from build123d import *

# Parameters (mm, degrees)
BOSS_EXTRUDE1_DEPTH      = 4.7625
M3_CLEARANCE_HOLE1_D     = 3.4
F_7_0_7_DIAMETER_HOLE1_D = 7
SKETCH12_R               = 11.5
CUT_EXTRUDE1_DEPTH       = 2.5


with BuildPart() as part:
    # Sketch1 → Boss-Extrude1 (new body)
    with BuildSketch(Plane(origin=(0, 0, 0), x_dir=(1, 0, 0), z_dir=(0, 1, 0))):
        Polygon((70, 65), (70, 45), (90, 45), (90, 0), (0, 0), (0, 65), align=None)
    extrude(amount=BOSS_EXTRUDE1_DEPTH)

    # M3 Clearance Hole1 (through all)
    with Locations(Plane(origin=(0, 4.7625, 0), x_dir=(1, 0, 0), z_dir=(0, 1, 0))):
        with Locations((36.709, 5.709), (36.709, 36.709), (5.709, 36.709), (5.709, 5.709)):
            Hole(M3_CLEARANCE_HOLE1_D / 2)

    # Ø7.0 (7) Diameter Hole1 (through all)
    with Locations(Plane(origin=(0, 0, 0), x_dir=(-1, 0, 0), z_dir=(0, -1, 0))):
        with Locations((-21.209, 21.209)):
            Hole(F_7_0_7_DIAMETER_HOLE1_D / 2)

    # Sketch12 → Cut-Extrude1 (cut)
    with BuildSketch(Plane.XZ):
        with Locations(Location((21.209, -21.209, 0), (0, 0, 270))):
            Circle(SKETCH12_R)
    extrude(amount=-CUT_EXTRUDE1_DEPTH, mode=Mode.SUBTRACT)


solid = part.part
Can you work these out from the model? Positions are in its coordinate system, mm. A direction names the side the tool comes from. Round coordinates to 2 decimals unless told otherwise and drop trailing zeros. Order: outer loops, then holes, each group sorted by start corner. A loop starts at its lowest first (then second) coordinate and runs counter-clockwise, first axis right, second up. Notation, with made-up numbers: (72, 44.5) - (102, 44.5) arc R27 ccw to (102, 63.5) - close; hole circle Ø2 at (-11, 39.25). An arc over 180 degrees is marked (long way). Answer in a Markdown table with one row per item.
(1) For P1, Ø11.5, axis at x = 17, z = -24, coming from the -Y side, with a flat end and sliding along its axis, tell me the tip position at first contact or that it passes through.
From the geometry:
| item | result |
|---|---|
| P1 | stops at y = 2.5 |
(2) Suppose I cut it at D-D, the plane z = -30. Please give me the cut outline in (x, y).
From the geometry:
| item | result |
|---|---|
| outline | (0, 0) - (13.79, 0) - (13.79, 2.5) - (28.62, 2.5) - (28.62, 0) - (90, 0) - (90, 4.76) - (0, 4.76) - close |
(3) Please list where these lines run through material, in increasing order: L1, parallel to X at y = 1.2, z = -21.5; L2, parallel to X at y = 3.95, z = -46; L3, parallel to Z at x = 76, y = 0.85. Write a range as from..to.
From the geometry:
| item | result |
|---|---|
| L1 | x = 0..9.71, 32.71..90 |
| L2 | x = 0..70 |
| L3 | z = -45..0 |
(4) Suppose I cut it at A-A, the plane x = 23. Please give me the cut outline in (y, z), plus the area to 3 significant figures.
From the geometry:
| item | result |
|---|---|
| outline | (0, -65) - (4.76, -65) - (4.76, -24.22) - (2.5, -24.22) - (2.5, -32.57) - (0, -32.57) - close; (0, -9.85) - (2.5, -9.85) - (2.5, -18.2) - (4.76, -18.2) - (4.76, 0) - (0, 0) - close |
| area | 239 mm2 |
(5) Suppose I cut it at C-C, the plane x = 37. Please give me the cut outline in (y, z).
From the geometry:
| item | result |
|---|---|
| outline | (0, -65) - (4.76, -65) - (4.76, -38.38) - (0, -38.38) - close; (0, -35.03) - (4.76, -35.03) - (4.76, -7.38) - (0, -7.38) - close; (0, -4.03) - (4.76, -4.03) - (4.76, 0) - (0, 0) - close |
(6) If we mould it in two halves opening along Z, with no side actions, what happens to faces 1 (the face through (24.442, 3.647, -19.868)), 2 (the face through (35, 2, -65)), 3 (the face through (90, 2, -23)), 4 (the face through (30.9, 1.2, -27.4))? For each: released by +Z, released by -Z, zero draft, split by the parting line, or undercut.
From the geometry:
| item | result |
|---|---|
| face 1 | undercut |
| face 2 | released by -Z |
| face 3 | zero draft |
| face 4 | undercut |
(7) Which directions (+Z, -Z, +X, -X, +Y, -Y) give clear straight access to the entire face, cutting with the end or side of a thin tool? Please do faces 5 (the face through (19, 2.5, -18)), 6 (the face through (0, 2, -32)), 7 (the face through (80, 2, -45)).
From the geometry:
| item | result |
|---|---|
| face 5 | -Y |
| face 6 | +Z, -Z, -X, +Y, -Y |
| face 7 | -Z, +X, +Y, -Y |
(8) Suppose I cut it at B-B, the plane y = 3.5. Please give me the cut outline in (x, z).
From the geometry:
| item | result |
|---|---|
| outline | (0, -65) - (70, -65) - (70, -45) - (90, -45) - (90, 0) - (0, 0) - close; hole circle Ø3.4 at (5.71, -36.71); hole circle Ø3.4 at (5.71, -5.71); hole circle Ø7 at (21.21, -21.21); hole circle Ø3.4 at (36.71, -36.71); hole circle Ø3.4 at (36.71, -5.71) |
